from build123d import *

# Parameters (mm, degrees)
F1_DEPTH      = 19.05
F1_DEPTH_BACK = 19.05
F2_SIZE       = 6.35
F3_W          = 50.8
F3_H          = 19.05
F4_DEPTH      = 38.101


with BuildPart() as f1:
    # F0 (on Front) → F1 (new body, two sides)
    with BuildSketch(Plane.XZ) as f1_sk:
        Polygon((1143, 95.25), (-1143, 95.25), (-1143, 44.45), (-1219.2, 44.45), (-1219.2, -44.45), (-1143, -44.45), (-1143, -95.25), (1143, -95.25), (1143, -44.45), (1219.2, -44.45), (1219.2, 44.45), (1143, 44.45), align=None)
    extrude(amount=F1_DEPTH)
    extrude(f1_sk.sketch, amount=-F1_DEPTH_BACK)

    # F2
    f2_edges = [f1.edges().sort_by_distance(p)[0] for p in [
        (1219.2, 0, 44.45),
        (1219.2, 0, -44.45),
        (-1219.2, 0, 44.45),
        (-1219.2, 0, -44.45),
    ]]
    chamfer(f2_edges, length=F2_SIZE)

    # F3 (on face) → F4 (cut, through all)
    with BuildSketch(Plane.XZ.offset(19.05)):
        with Locations((1168.4, 0)):
            Rectangle(F3_W, F3_H)
        with Locations((-1168.4, 0)):
            Rectangle(F3_W, F3_H)
    extrude(amount=-F4_DEPTH, mode=Mode.SUBTRACT)


solid = f1.part
Geometry check sheet. Reference: the model listing, model coordinates, mm. A direction names the side the tool comes from. Round coordinates to 2 decimals unless told otherwise and drop trailing zeros. Loops run counter-clockwise (first coordinate to the right, second up) from the corner with the lowest first, then second, coordinate; pieces in that order, holes last. Notation, with made-up numbers: (63.5, -13.5) - (88.5, -13.5) arc R26 cw to (88.5, 11.5) - close; hole circle Ø1 at (80.25, 6). An arc over 180 degrees is marked (long way). One line per question, with ' | ' between items. Start each with the question number.
1. Cross-section at A-A on y = -9.5. Record the cut outline in (x, z) (3 decimals).
2. Tool access check on faces 1 (the face through (1168, 0, -9.525)), 2 (the face through (1143, 0, -70)), 3 (the face through (-1143, 0, 70)), 4 (the face through (-1178, 0, -44.45)). Record the directions out of +Z, -Z, +X, -X, +Y, -Y that give a thin tool (end or side, any length) a straight path to the whole face; none if there is none.
3. Scan lines: line 1 (X direction, y = 1, z = -4); line 2 (X direction, y = 6.5, z = 66); line 3 (X direction, y = -11, z = 38.5). Record each from-to range of solid material in increasing order. Write a range as [from, to].
4. Cross-section at B-B on z = 72. Record the cut outline in (x, y).
5. Depth check by flat-ended pin: pin 1 (11.5 mm diameter, centred on x = 1167.5, y = 4, fed in from +Z); pin 2 (11.5 mm diameter, centred on y = -9.5, z = -63, fed in from +X). Enter the tip coordinate at first touch or a pass-through.
Taken from the geometry:
1) outline: (-1219.2, -38.1) - (-1212.85, -44.45) - (-1143, -44.45) - (-1143, -95.25) - (1143, -95.25) - (1143, -44.45) - (1212.85, -44.45) - (1219.2, -38.1) - (1219.2, 38.1) - (1212.85, 44.45) - (1143, 44.45) - (1143, 95.25) - (-1143, 95.25) - (-1143, 44.45) - (-1212.85, 44.45) - (-1219.2, 38.1) - close; hole (-1193.8, -9.525) - (-1143, -9.525) - (-1143, 9.525) - (-1193.8, 9.525) - close; hole (1143, -9.525) - (1193.8, -9.525) - (1193.8, 9.525) - (1143, 9.525) - close
2) face 1: +Y, -Y | face 2: -Z, +X, +Y, -Y | face 3: +Z, -X, +Y, -Y | face 4: -Z, -X, +Y, -Y
3) line 1: [-1219.2, -1193.8], [-1143, 1143], [1193.8, 1219.2] | line 2: [-1143, 1143] | line 3: [-1218.8, 1218.8]
4) outline: (-1143, -19.05) - (1143, -19.05) - (1143, 19.05) - (-1143, 19.05) - close
5) pin 1: z = 44.45 | pin 2: x = 1143
